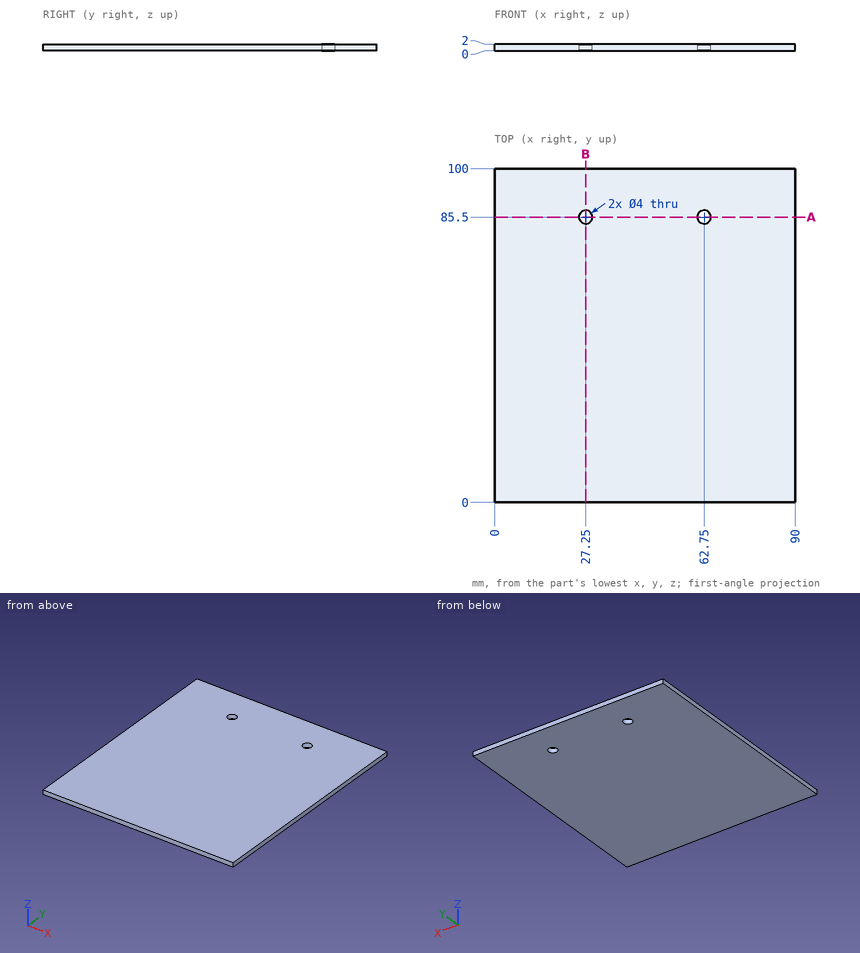
Input: dimensioned drawing with shaded views. Units: mm. Origin: part minimum x, y, z. Round coordinates to 2 decimals unless told otherwise and drop trailing zeros. Order: outer loops, then holes, each group sorted by start corner. A loop starts at its lowest first (then second) coordinate and runs counter-clockwise, first axis right, second up.
1. Cut plane A-A, the plane y = 85.5. Output: boundary loops of the cut face in (x, z), then the cut area to 3 significant figures.
The answers:
outline: (0, 0) - (25.25, 0) - (25.25, 2) - (0, 2) - close; (29.25, 0) - (60.75, 0) - (60.75, 2) - (29.25, 2) - close; (64.75, 0) - (90, 0) - (90, 2) - (64.75, 2) - close
area: 164 mm2
2. Pin query (flat end, axial travel): P1, Ø3, axis at x = 20.5, y = 73, coming from the -Z side. Return the tip coordinate at first contact, or that it passes through.
The answers:
P1: stops at z = 0
3. Cut plane B-B, the plane x = 27.25. Output: boundary loops of the cut face in (y, z), then the cut area to 3 significant figures.
The answers:
outline: (0, 0) - (83.5, 0) - (83.5, 2) - (0, 2) - close; (87.5, 0) - (100, 0) - (100, 2) - (87.5, 2) - close
area: 192 mm2
4. Material intervals for line 1 (Y direction, x = 27.25, z = 0.7); line 2 (X direction, y = 86, z = 1.5); line 3 (Y direction, x = 28.5, z = 0.3), sorted ascending.
The answers:
line 1: y = 0 to 83.5, 87.5 to 100
line 2: x = 0 to 25.31, 29.19 to 60.81, 64.69 to 90
line 3: y = 0 to 83.94, 87.06 to 100
